CAD build for the part. Positions are in the model's coordinates, mm. Face numbers are marked on the shaded views. A direction names the side the tool comes from. Give positions to 0.01 mm unless a question says otherwise; leave off trailing zeros. Order: outer loops, then holes, each group sorted by start corner. A loop starts at its lowest first (then second) coordinate and runs counter-clockwise, first axis right, second up.
from build123d import *

# Parameters (mm, degrees)
BOX_EXTRUDE_PART_DEPTH         = 80
BOX_EXTRUDE_PART_DEPTH_BACK    = 15
BOX_TOP_VIEW_W                 = 140
BOX_TOP_VIEW_H                 = 120
INNER_BOX_CUT_W                = 120
INNER_BOX_CUT_H                = 100
INNER_BOX_CUT_1_DEPTH          = 40
SCISSOR_CROSSSECTION_W         = 115
SCISSOR_CROSSSECTION_H         = 10
SCISSOR_CORSSSECTION_CUT_DEPTH = 10
SHAFT_LOCATION_R               = 6
SHAFT_LOCATION_CUT_DEPTH       = 40
SKETCH2_R                      = 16
SKETCH2_R_2                    = 8
BEARING_LOCATION_CUT1_DEPTH    = 10
M6_TAPPED_HOLE3_AT_2_COUNT     = 2
M6_TAPPED_HOLE3_AT_2_PITCH     = 85.14693183
EDGES_FILLET_R                 = 4


with BuildPart() as part:
    # Box_top_view → Box_extrude_part (new, two sides: drawn at the far end of the back side and taken through both)
    with BuildSketch(Plane(origin=(0, 0, 0), x_dir=(1, 0, 0), z_dir=(0, 1, 0)).offset(-BOX_EXTRUDE_PART_DEPTH_BACK)):
        Rectangle(BOX_TOP_VIEW_W, BOX_TOP_VIEW_H)
    extrude(amount=BOX_EXTRUDE_PART_DEPTH + BOX_EXTRUDE_PART_DEPTH_BACK)

    # Inner_box_cut → Inner_box_cut_1 (cut)
    with BuildSketch(Plane(origin=(0, 80, 0), x_dir=(1, 0, 0), z_dir=(0, 1, 0))):
        Rectangle(INNER_BOX_CUT_W, INNER_BOX_CUT_H)
    extrude(amount=-INNER_BOX_CUT_1_DEPTH, mode=Mode.SUBTRACT)

    # Scissor_crossSection → Scissor_corssSection_cut (cut)
    with BuildSketch(Plane.XY.offset(60)):
        with Locations((0, 50)):
            Rectangle(SCISSOR_CROSSSECTION_W, SCISSOR_CROSSSECTION_H)
    extrude(amount=-SCISSOR_CORSSSECTION_CUT_DEPTH, mode=Mode.SUBTRACT)

    # Shaft_location → Shaft_location_cut (cut)
    with BuildSketch(Plane(origin=(0, 40, 0), x_dir=(1, 0, 0), z_dir=(0, 1, 0))):
        with Locations(Location((15, 0, 0), (0, 0, 270))):
            Circle(SHAFT_LOCATION_R)
        with Locations(Location((-15, 0, 0), (0, 0, 90))):
            Circle(SHAFT_LOCATION_R)
    extrude(amount=-SHAFT_LOCATION_CUT_DEPTH, mode=Mode.SUBTRACT)

    # Sketch2 → Bearing_location_cut1 (cut)
    with BuildSketch(Plane(origin=(0, 40, 0), x_dir=(1, 0, 0), z_dir=(0, 1, 0))):
        with Locations(Location((-15, 0, 0), (0, 0, 270))):
            Circle(SKETCH2_R)
        with Locations(Location((15, 0, 0), (0, 0, 90))):
            Circle(SKETCH2_R_2)
    extrude(amount=-BEARING_LOCATION_CUT1_DEPTH, mode=Mode.SUBTRACT)

    # Sketch7 → M6 Tapped Hole3 (revolve, cut)
    with BuildSketch(Plane(origin=(0, 80, -55), x_dir=(0, 0, 1), z_dir=(1, 0, 0))):
        Polygon((0, 0), (0, 14.502151548), (2.5, 13), (2.5, 0.525), (3.025, 0), align=None)
    m6_tapped_hole3 = revolve(axis=Axis((0, 86.35, -55), (0, -1, 0)), mode=Mode.SUBTRACT)

    # M6 Tapped Hole3 at 2: M6 Tapped Hole3 ×2
    with Locations(*[Vector(-0.7633862853691146, 0, 0.645942241466174) * (i * M6_TAPPED_HOLE3_AT_2_PITCH) for i in range(1, M6_TAPPED_HOLE3_AT_2_COUNT)]):
        add(m6_tapped_hole3, mode=Mode.SUBTRACT)

    # M6_hole_mirror: M6 Tapped Hole3 across plane
    add(m6_tapped_hole3.mirror(Plane(origin=(0, 0, 0), x_dir=(0, 0, 1), z_dir=(1, 0, 0))), mode=Mode.SUBTRACT)

    # M6_hole_mirror copy 1 sketch → M6_hole_mirror copy 1 (revolve, cut)
    with BuildSketch(Plane(origin=(65, 80, 0), x_dir=(0, 0, 1), z_dir=(-1, 0, 0))):
        Polygon((0, 0), (0, -14.502151548), (2.5, -13), (2.5, -0.525), (3.025, 0), align=None)
    revolve(axis=Axis((65, 86.35, 0), (0, 1, 0)), mode=Mode.SUBTRACT)

    # M6_hole_mirror at the second plane: M6 Tapped Hole3 across plane
    add(m6_tapped_hole3.mirror(Plane.XY), mode=Mode.SUBTRACT)

    # M6_hole_mirror at the second plane copy → M6_hole_mirror at the second plane c 2 (revolve, cut)
    with BuildSketch(Plane(origin=(-65, 80, 0), x_dir=(0, 0, -1), z_dir=(1, 0, 0))):
        Polygon((0, 0), (0, -14.502151548), (2.5, -13), (2.5, -0.525), (3.025, 0), align=None)
    revolve(axis=Axis((-65, 86.35, 0), (0, 1, 0)), mode=Mode.SUBTRACT)

    # Edges_fillet
    edges_fillet_edges = [part.edges().sort_by_distance(p)[0] for p in [
        (70, -15, 0),
        (0, -15, -60),
        (-70, -15, 0),
        (-70, 32.5, -60),
        (70, 32.5, -60),
        (70, 32.5, 60),
        (-70, 32.5, 60),
        (0, -15, 60),
    ]]
    fillet(edges_fillet_edges, radius=EDGES_FILLET_R)


solid = part.part
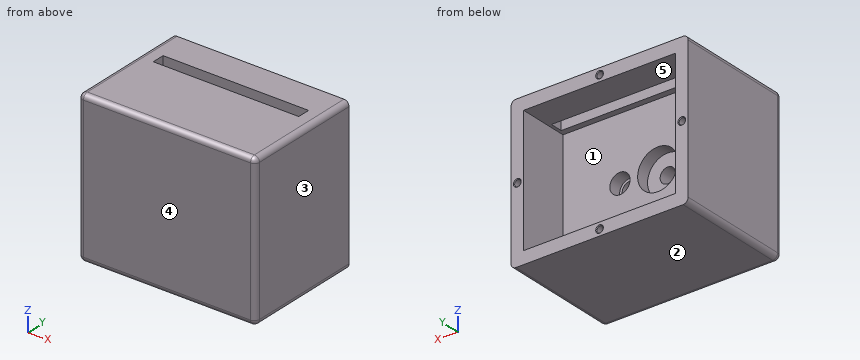
1. Saw through at A-A on x = -15. Give the cut face in (y, z).
2. Saw through at C-C on z = -43. Give the cut face in (x, y), plus the area to 3 significant figures.
3. Wall check: line 1 (Z direction, x = 0, y = 74); line 2 (X direction, y = 68.5, z = 10); line 3 (Z direction, x = -65, y = 77.25). Give the ranges that are in metal, low to high.
4. Mould opens along X. For the marked faces 1, 2 and 3 say: released by +X, released by -X, zero draft, split by the parting line, or undercut.
5. Saw through at B-B on y = 60. Give the cut face in (x, z).
6. Saw through at D-D on x = 39.5. Give the cut face in (y, z), plus the area to 3 significant figures.
7. 3-axis set-ups, long thin cutter, end or side, ignore diameter. For the marked faces 4 and 5: which of +Z, -Z, +X, -X, +Y, -Y reach the whole face in a straight line?
8. Pin check, flat tips, straight feed: P1, Ø3.5, axis at x = 17.5, z = -3, coming from the +Y side; P2, Ø13, axis at x = 18, z = -2.5, coming from the +Y side; P3, Ø4, axis at x = 0, z = -55, coming from the +Y side. Stop position of each tip, or through.
Reported:
1. outline: (-15, -56) arc R4 ccw to (-11, -60) - (80, -60) - (80, -50) - (40, -50) - (40, -16) - (30, -16) - (30, -6) - (0, -6) - (0, 6) - (30, 6) - (30, 16) - (40, 16) - (40, 50) - (45, 50) - (45, 60) - (-11, 60) arc R4 ccw to (-15, 56) - close; (55, 50) - (80, 50) - (80, 60) - (55, 60) - close
2. outline: (-70, -11) arc R4 ccw to (-66, -15) - (66, -15) arc R4 ccw to (70, -11) - (70, 80) - (60, 80) - (60, 40) - (-60, 40) - (-60, 80) - (-70, 80) - close
2. area: 8,490 mm2
3. line 1: z = -60 to -57.5, -52.5 to -50, 50 to 52.5, 57.5 to 60
3. line 2: x = -70 to -60, 60 to 70
3. line 3: z = -60 to -2.5, 2.5 to 60
4. face 1: undercut
4. face 2: zero draft
4. face 3: released by +X
5. outline: (-70, -56) arc R4 ccw to (-66, -60) - (66, -60) arc R4 ccw to (70, -56) - (70, 56) arc R4 ccw to (66, 60) - (-66, 60) arc R4 ccw to (-70, 56) - close; hole (-60, -50) - (60, -50) - (60, 50) - (-60, 50) - close
6. outline: (-15, -56) arc R4 ccw to (-11, -60) - (80, -60) - (80, -50) - (40, -50) - (40, 50) - (45, 50) - (45, 60) - (-11, 60) arc R4 ccw to (-15, 56) - close; (55, 50) - (80, 50) - (80, 60) - (55, 60) - close
6. area: 7,290 mm2
7. face 4: +Z, -Z, +X, -X, -Y
7. face 5: +Y
8. P1: stops at y = 0
8. P2: stops at y = 40
8. P3: stops at y = 66.7
